CAD build for the part. Positions are in the model's coordinates, mm. Round coordinates to 2 decimals unless told otherwise and drop trailing zeros. Order: outer loops, then holes, each group sorted by start corner. A loop starts at its lowest first (then second) coordinate and runs counter-clockwise, first axis right, second up. Notation, with made-up numbers: M 17,-13.5 L 29,-13.5 A23 cw 29,6.5 Z; hole C 2.25,79.5 d10. An arc over 180 degrees is marked long. Answer as a JSON object with one key per item and string values.
```python
from build123d import *

# Parameters (mm, degrees)
F2_R     = 2.5
F3_DEPTH = 6
F4_DEPTH = 25


with BuildPart() as f1:
    # F0 (on Front) → F1 (revolve)
    with BuildSketch(Plane.XZ):
        Polygon((-4.375, 0), (-2, 0), (-2, 18.5), (-4.375, 18.5), (-4.375, 2), (-13.835, 2), (-13.835, 0), align=None)
    revolve(axis=Axis((0, 0, 9.25), (0, 0, 1)))

    # F2 (on face) → F3 (join)
    with BuildSketch(Plane.XY.offset(2)):
        with BuildLine():
            ThreePointArc((-4.328894081, -0.6334832559), (-4.375, 0), (-4.328894081, 0.6334832559))
            ThreePointArc((-4.328894081, 0.6334832559), (-11.775, 0), (-4.328894081, -0.6334832559))
        make_face()
        with Locations((-8.025, 0)):
            Circle(F2_R, mode=Mode.SUBTRACT)
        with BuildLine():
            ThreePointArc((11.775, 0), (8.3428858315, 3.7365021876), (4.328894081, 0.6334832559))
            ThreePointArc((4.328894081, 0.6334832559), (4.3634582961, 0.3175794354), (4.375, 0))
            ThreePointArc((4.375, 0), (4.3634582961, -0.3175794354), (4.328894081, -0.6334832559))
            ThreePointArc((4.328894081, -0.6334832559), (8.3428858315, -3.7365021876), (11.775, 0))
        make_face()
        with Locations((8.025, 0)):
            Circle(F2_R, mode=Mode.SUBTRACT)
    extrude(amount=F3_DEPTH)

    # F4 (cut): faces of the model
    f4_faces = [f1.faces().sort_by_distance(p)[0] for p in [
        (-8.025, 0, 2),
        (8.025, 0, 2),
    ]]
    extrude(f4_faces, amount=-F4_DEPTH, mode=Mode.SUBTRACT)


solid = f1.part
```
Item 1: Saw through at A-A on x = 0. List the corners of the cut face in (y, z) (3 decimals).
Worked answers:
{"outline": "M -13.835,0 L -2,0 L -2,18.5 L -4.375,18.5 L -4.375,2 L -13.835,2 Z; M 2,0 L 13.835,0 L 13.835,2 L 4.375,2 L 4.375,18.5 L 2,18.5 Z"}
Item 2: Saw through at B-B on z = 4.5. List the corners of the cut face in (x, y) (3 decimals), and give its area (3 significant figures).
Worked answers:
{"outline": "M -4.329,-0.633 A4.375 ccw 4.329,-0.633 A3.75 ccw long 4.329,0.633 A4.375 ccw -4.329,0.633 A3.75 ccw long Z; hole C -8.025,0 d5; hole C 0,0 d4; hole C 8.025,0 d5", "area": "96.5 mm2"}
Item 3: Wall check: line 1 along Z through (x, y) = (-4.75, 6); line 2 along Y through (x, z) = (0, 7.5) (3 decimals); line 3 along Y through (x, z) = (6, 6.75). Give the ranges that are in metal, low to high. Write a range as [from, to].
Worked answers:
{"line 1": "z = [0, 2]", "line 2": "y = [-4.375, -2], [2, 4.375]", "line 3": "y = [-3.16, -1.47], [1.47, 3.16]"}
Item 4: Two-plate mould, pull along Y, no slides. Class faces 1 (the flat face through (-8, 3, 8)), 2 (the cylindrical face through (0, 2, 9)), 3 (the cylindrical face through (13.82, -0.61, 0.99)): released by +Y, released by -Y, zero draft, split by the parting line, or undercut.
Worked answers:
{"face 1": "zero draft", "face 2": "undercut", "face 3": "split by the parting line"}
Item 5: Saw through at C-C on x = -6. List the corners of the cut face in (y, z), and give its area (3 significant figures).
Worked answers:
{"outline": "M -12.47,0 L -1.47,0 L -1.47,8 L -3.16,8 L -3.16,2 L -12.47,2 Z; M 1.47,0 L 12.47,0 L 12.47,2 L 3.16,2 L 3.16,8 L 1.47,8 Z", "area": "64.3 mm2"}
Item 6: Saw through at D-D on z = 11.75. List the corners of the cut face in (x, y) (3 decimals).
Worked answers:
{"outline": "C 0,0 d8.75; hole C 0,0 d4"}
Item 7: Drop flat-ended pins along their axis: pin 1 Ø1 at (y, z) = (1, 3.5) entering from +X; pin 2 Ø10 at (x, y) = (-6, 7.5) entering from +Z; pin 3 Ø1 at (x, y) = (3, 4.5) entering from +Z; pin 4 Ø4 at (x, y) = (-8.025, 0) entering from -Z. Give the stop position or say it passes through.
Worked answers:
{"pin 1": "stops at x = 11.74", "pin 2": "stops at z = 8", "pin 3": "stops at z = 2", "pin 4": "passes through"}
